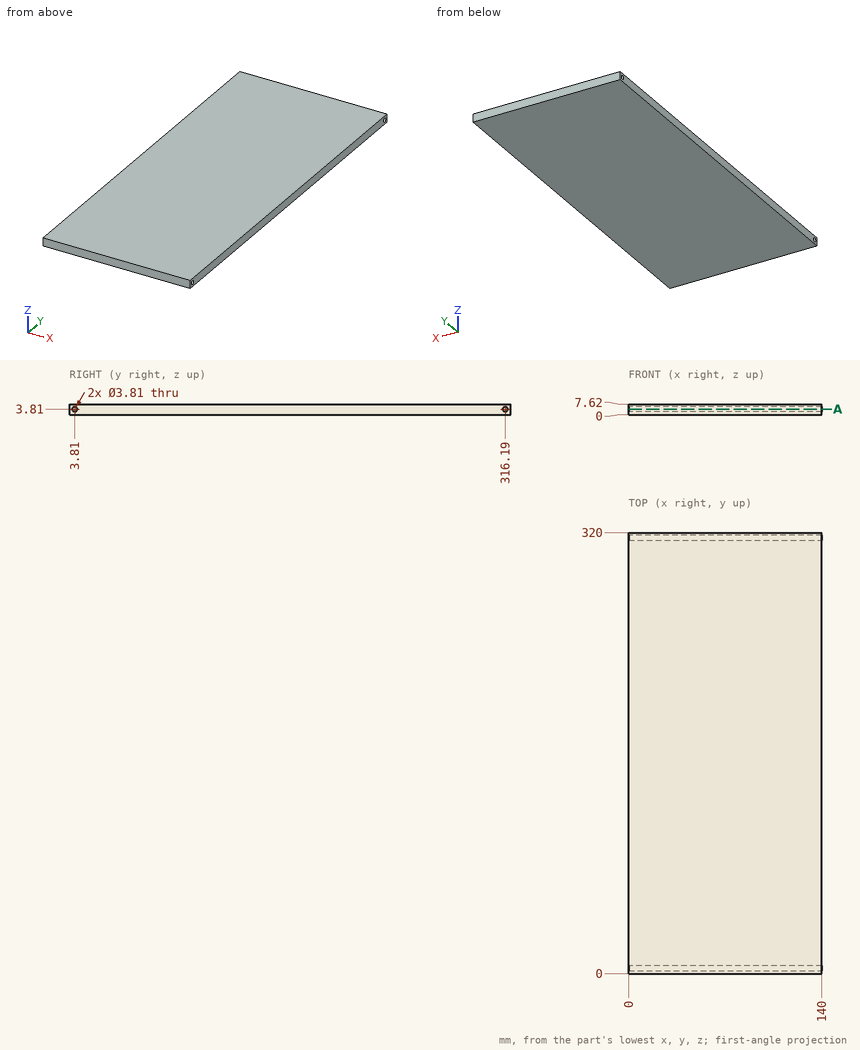
Answer from the drawing. Dimensions are ordinates in mm from the lowest x, y and z of the part. Round coordinates to 2 decimals unless told otherwise and drop trailing zeros. Write each loop counter-clockwise with the first axis right and the second up, starting at its lowest first coordinate (ties: lowest second). Pieces come first, ordered by that corner, then holes. Notation, with made-up numbers: (11, 67.5) -> (66, 67.5) arc R35 ccw to (66, 102.5) -> close; hole circle Ø10 at (-37.75, -37.5). An arc over 180 degrees is marked (long way). Answer in a Markdown table with one row per item. Add a question column.
1) Given P1, Ø1, axis at x = 73, z = 5.5, coming from the -Y side, flat-ended and moving along its own axis, determine where the tip first touches the part or whether it passes through.
2) Consider line 1 (Z direction, x = 42, y = 3.81) (3 decimals); line 2 (Y direction, x = 31, z = 2.75); line 3 (Y direction, x = 16.5, z = 5.25). Determine where each line is inside the solid, lowest interval first.
3) Find section A-A, the plane z = 3.81. Determine the outline of the cut face in (x, y) (3 decimals).
Findings below:
| question | item | result |
|---|---|---|
| 1 | P1 | y = 0 |
| 2 | line 1 | 0 to 1.905, 5.715 to 7.62 |
| 2 | line 2 | 0 to 2.23, 5.39 to 314.61, 317.77 to 320 |
| 2 | line 3 | 0 to 2.56, 5.06 to 314.94, 317.44 to 320 |
| 3 | outline | (0, 0) -> (140, 0) -> (140, 1.905) -> (0, 1.905) -> close; (0, 5.715) -> (140, 5.715) -> (140, 314.285) -> (0, 314.285) -> close; (0, 318.095) -> (140, 318.095) -> (140, 320) -> (0, 320) -> close |
